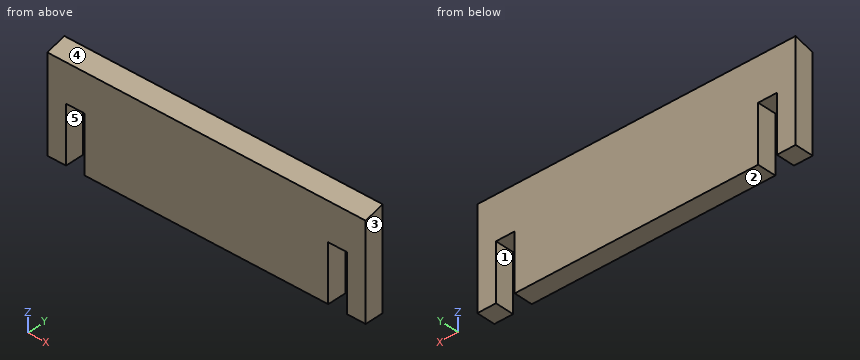
```python
from build123d import *

# Parameters (mm, degrees)
BOSS_EXTRUDE1_DEPTH = 10
DRAFT2_ANGLE        = 15


with BuildPart() as part:
    # Sketch1 → Boss-Extrude1 (new body)
    with BuildSketch(Plane(origin=(0, 0, 0), x_dir=(1, 0, 0), z_dir=(0, 1, 0))):
        Polygon((-75, 25), (-75, -5), (-65, -5), (-65, 25), (65, 25), (65, -5), (75, -5), (75, 25), (85, 25), (85, -25), (-85, -25), (-85, 25), align=None)
    extrude(amount=BOSS_EXTRUDE1_DEPTH)

    # Draft2
    draft2_faces = [part.faces().sort_by_distance(p)[0] for p in [
        (0, 5, 25),
    ]]
    draft(draft2_faces, Plane(origin=(0, 0, 0), x_dir=(0, 0, -1), z_dir=(0, -1, 0)), DRAFT2_ANGLE)


solid = part.part
```
Geometry check sheet. Reference: the model listing, model coordinates, mm. Face numbers are marked on the shaded views. A direction names the side the tool comes from. Coordinates: 2 decimals unless noted, no trailing zeros. Write each loop counter-clockwise with the first axis right and the second up, starting at its lowest first coordinate (ties: lowest second). Pieces come first, ordered by that corner, then holes. Notation, with made-up numbers: (49.25, 1.5) -> (82.25, 1.5) arc R18 cw to (82.25, 15.5) -> close; hole circle Ø5 at (-39, 33). An arc over 180 degrees is marked (long way). Use CSV: the item, a comma, the result in double quotes. Start each with the question number.
Item 1: Set-up check for the marked faces 1 and 2: record each of +Z, -Z, +X, -X, +Y, -Y from which the full face is reachable in a straight line by a thin tool's end or side.
Item 2: Cross-section at D-D, the plane x = -32.5. Record the cut outline in (y, z), plus the area to 3 significant figures.
Item 3: Cross-section at A-A, the plane z = -11. Record the cut outline in (x, y).
Item 4: Mould release check, pull along X, two halves, no side actions. Record for the marked faces 3, 4 and 5: released by +X, released by -X, zero draft, split by the parting line, or undercut.
Item 5: Cross-section at B-B, the plane y = 4.75. Record the cut outline in (x, z), plus the area to 3 significant figures.
Item 6: Thickness scan on line 1 (X direction, y = 7.75, z = -1.5); line 2 (Z direction, x = 37.5, y = 8.5); line 3 (Z direction, x = 61.5, y = 4). Record the ranges inside material, lowest first.
Item 7: Depth check by flat-ended pin: pin 1 Ø2 at (x, y) = (-46, 5.5) entering from +Z; pin 2 Ø2 at (x, y) = (9.5, 7) entering from +Z. Enter the tip coordinate at first touch or a pass-through.
Item 8: Cross-section at C-C, the plane x = 68.5. Record the cut outline in (y, z).
Answers:
1,face 1,"-Z, +Y, -Y"
1,face 2,"-Z, +X, -X, +Y, -Y"
2,outline,"(0, -25) -> (10, -25) -> (10, 27.68) -> (0, 25) -> close"
2,area,"513 mm^2"
3,outline,"(-85, 0) -> (-75, 0) -> (-75, 10) -> (-85, 10) -> close; (-65, 0) -> (65, 0) -> (65, 10) -> (-65, 10) -> close; (75, 0) -> (85, 0) -> (85, 10) -> (75, 10) -> close"
4,face 3,"released by +X"
4,face 4,"zero draft"
4,face 5,"undercut"
5,outline,"(-85, -25) -> (-75, -25) -> (-75, 5) -> (-65, 5) -> (-65, -25) -> (65, -25) -> (65, 5) -> (75, 5) -> (75, -25) -> (85, -25) -> (85, 26.27) -> (-85, 26.27) -> close"
5,area,"8,120 mm^2"
6,line 1,"-85 to -75, -65 to 65, 75 to 85"
6,line 2,"-25 to 27.28"
6,line 3,"-25 to 26.07"
7,pin 1,"z = 26.74"
7,pin 2,"z = 27.14"
8,outline,"(0, 5) -> (10, 5) -> (10, 27.68) -> (0, 25) -> close"
